Input: part model. Units: mm. Frame: model coordinates. A direction names the side the tool comes from. Round coordinates to 2 decimals unless told otherwise and drop trailing zeros. Order: outer loops, then holes, each group sorted by start corner. A loop starts at its lowest first (then second) coordinate and runs counter-clockwise, first axis right, second up. Notation, with made-up numbers: (89, 54.5) - (97, 54.5) arc R18 ccw to (97, 78.5) - close; hole circle Ø10 at (43.25, 60.5). An arc over 180 degrees is marked (long way). One line per item, written item: value. Start each with the question number.
from build123d import *

# Parameters (mm, degrees)
BOSS_EXTRUDE1_DEPTH   = 29
BOSS_EXTRUDE1_2_DEPTH = 29
FILLET1_R             = 1
FILLET2_R             = 1
SKETCH3_R             = 10
BOSS_EXTRUDE2_DEPTH   = 26.527316462
SKETCH4_R             = 2.5
CUT_EXTRUDE4_DEPTH    = 112.4075373


with BuildPart() as part:
    # Sketch1 → Boss-Extrude1 (new body)
    with BuildSketch(Plane.XY):
        with BuildLine():
            Line((-12.418786495, 106.527316462), (12.418786495, 106.527316462))
            ThreePointArc((12.418786495, 106.527316462), (14.186553448, 105.795083415), (14.918786495, 104.027316462))
            Line((14.918786495, 104.027316462), (14.918786495, 69.027316462))
            ThreePointArc((14.918786495, 69.027316462), (14.186553448, 67.259549509), (12.418786495, 66.527316462))
            Line((12.418786495, 66.527316462), (7.418786495, 66.527316462))
            Line((7.418786495, 66.527316462), (-7.418786495, 66.527316462))
            Line((-7.418786495, 66.527316462), (-12.418786495, 66.527316462))
            ThreePointArc((-12.418786495, 66.527316462), (-14.186553448, 67.259549509), (-14.918786495, 69.027316462))
            Line((-14.918786495, 69.027316462), (-14.918786495, 104.027316462))
            ThreePointArc((-14.918786495, 104.027316462), (-14.186553448, 105.795083415), (-12.418786495, 106.527316462))
        make_face()
    extrude(amount=BOSS_EXTRUDE1_DEPTH)

    # Fillet2
    fillet2_edges = [part.edges().sort_by_distance(p)[0] for p in [
        (14.186553448, 105.795083415, 0),
        (0, 106.527316462, 0),
        (-14.186553448, 105.795083415, 0),
        (-14.918786495, 86.527316462, 0),
        (-14.186553448, 67.259549509, 0),
        (0, 66.527316462, 0),
        (14.186553448, 67.259549509, 0),
        (14.918786495, 86.527316462, 0),
        (14.186553448, 105.795083415, 29),
        (0, 106.527316462, 29),
        (-14.186553448, 105.795083415, 29),
        (-14.918786495, 86.527316462, 29),
        (-14.186553448, 67.259549509, 29),
        (0, 66.527316462, 29),
        (14.186553448, 67.259549509, 29),
        (14.918786495, 86.527316462, 29),
    ]]
    fillet(fillet2_edges, radius=FILLET2_R)



with BuildPart() as body_2:
    # Sketch1 → Boss-Extrude1 2 (new body)
    with BuildSketch(Plane.XY):
        with BuildLine():
            Line((7.418786495, 40), (12.418786495, 40))
            ThreePointArc((12.418786495, 40), (14.186553448, 39.267766953), (14.918786495, 37.5))
            Line((14.918786495, 37.5), (14.918786495, -2.5))
            ThreePointArc((14.918786495, -2.5), (14.186553448, -4.267766953), (12.418786495, -5))
            Line((12.418786495, -5), (-12.418786495, -5))
            ThreePointArc((-12.418786495, -5), (-14.186553448, -4.267766953), (-14.918786495, -2.5))
            Line((-14.918786495, -2.5), (-14.918786495, 37.5))
            ThreePointArc((-14.918786495, 37.5), (-14.186553448, 39.267766953), (-12.418786495, 40))
            Line((-12.418786495, 40), (-7.418786495, 40))
            Line((-7.418786495, 40), (7.418786495, 40))
        make_face()
    extrude(amount=BOSS_EXTRUDE1_2_DEPTH)

    # Fillet1
    fillet1_edges = [body_2.edges().sort_by_distance(p)[0] for p in [
        (-14.918786495, 17.5, 0),
        (-14.186553448, 39.267766953, 0),
        (0, 40, 0),
        (14.186553448, 39.267766953, 0),
        (14.918786495, 17.5, 0),
        (14.186553448, -4.267766953, 29),
        (14.186553448, -4.267766953, 0),
        (0, -5, 0),
        (-14.186553448, -4.267766953, 0),
        (14.918786495, 17.5, 29),
        (14.186553448, 39.267766953, 29),
        (0, 40, 29),
        (-14.186553448, 39.267766953, 29),
        (-14.918786495, 17.5, 29),
        (-14.186553448, -4.267766953, 29),
        (0, -5, 29),
    ]]
    fillet(fillet1_edges, radius=FILLET1_R)


with BuildPart() as part_1:
    add(part.part)

    add(body_2.part)  # Boss-Extrude2 merges body 2
    # Sketch3 → Boss-Extrude2 (add)
    with BuildSketch(Plane(origin=(0, 40, 0), x_dir=(1, 0, 0), z_dir=(0, 1, 0))):
        with Locations(Location((0, -14.5, 0), (0, 0, 90))):
            Circle(SKETCH3_R)
    extrude(amount=BOSS_EXTRUDE2_DEPTH)

    # Sketch4 → Cut-Extrude4 (cut, through all)
    with BuildSketch(Plane(origin=(0, 0, 0), x_dir=(-1, 0, 0), z_dir=(0, 0, -1))):
        with Locations((0, 97.5)):
            Circle(SKETCH4_R)
        with Locations((0, 2.5)):
            Circle(SKETCH4_R)
    extrude(amount=-CUT_EXTRUDE4_DEPTH, mode=Mode.SUBTRACT)


solid = part_1.part
1. Section A-A (z = 26.25). Return the cut outline in (x, y), then the cut area to 3 significant figures.
2. Line query: line 1 (Y direction, x = 0, z = 15.25); line 2 (Y direction, x = -9.75, z = 9.75); line 3 (Y direction, x = -1.75, z = 11.75). Output: solid intervals per line, ascending. Write a range as from..to.
3. Section C-C (x = 0). Return the cut outline in (y, z).
4. Pull-direction query (Y, two-part tool) for faces 1 (the face through (-14.167, -4.287, 14.311)), 2 (the face through (-14.919, 86, 14)), 3 (the face through (-3, 53.08, 4.96)); classes: released by +Y, released by -Y, zero draft, split by the parting line, or undercut.
5. Set-up query: faces 4 (the face through (-14.206, 39.248, 14.311)), 5 (the face through (14.206, 67.279, 14.311)), 6 (the face through (8, 66.527, 8)). Return all of +Z, -Z, +X, -X, +Y, -Y with unobstructed straight access to the full face (end or side cutting, diameter ignored); none if empty.
6. Section D-D (z = 14.5). Return the cut outline in (x, y).
7. Pin query (flat end, axial travel): pin 1 (3 mm diameter, centred on y = 60.5, z = 8, fed in from -X); pin 2 (5 mm diameter, centred on y = 60, z = 17, fed in from -X); pin 3 (3 mm diameter, centred on x = 0, y = 2.5, fed in from -Z); pin 4 (5 mm diameter, centred on x = -0.5, y = 54, fed in from -Z). Return the tip coordinate at first contact, or that it passes through.
8. Section B-B (y = 2.5). Return the cut outline in (x, z), then the cut area to 3 significant figures.
Solved:
1. outline: (-14.92, -2.5) arc R2.5 ccw to (-12.42, -5) - (12.42, -5) arc R2.5 ccw to (14.92, -2.5) - (14.92, 37.5) arc R2.5 ccw to (12.42, 40) - (-12.42, 40) arc R2.5 ccw to (-14.92, 37.5) - close; (-14.92, 69.03) arc R2.5 ccw to (-12.42, 66.53) - (12.42, 66.53) arc R2.5 ccw to (14.92, 69.03) - (14.92, 104.03) arc R2.5 ccw to (12.42, 106.53) - (-12.42, 106.53) arc R2.5 ccw to (-14.92, 104.03) - close; hole circle Ø5 at (0, 2.5); hole circle Ø5 at (0, 97.5)
1. area: 2,490 mm²
2. line 1: y = -5..0, 5..95, 100..106.53
2. line 2: y = -5..40, 66.53..106.53
2. line 3: y = -5..0.71, 4.29..95.71, 99.29..106.53
3. outline: (-5, 1) arc R1 ccw to (-4, 0) - (0, 0) - (0, 29) - (-4, 29) arc R1 ccw to (-5, 28) - close; (5, 0) - (39, 0) arc R1 ccw to (40, 1) - (40, 4.5) - (66.53, 4.5) - (66.53, 1) arc R1 ccw to (67.53, 0) - (95, 0) - (95, 29) - (67.53, 29) arc R1 ccw to (66.53, 28) - (66.53, 24.5) - (40, 24.5) - (40, 28) arc R1 ccw to (39, 29) - (5, 29) - close; (100, 0) - (105.53, 0) arc R1 ccw to (106.53, 1) - (106.53, 28) arc R1 ccw to (105.53, 29) - (100, 29) - close
4. face 1: released by -Y
4. face 2: zero draft
4. face 3: undercut
5. face 4: +Z, -Z, -X
5. face 5: +Z, -Z, +X
5. face 6: none
6. outline: (-14.92, -2.5) arc R2.5 ccw to (-12.42, -5) - (12.42, -5) arc R2.5 ccw to (14.92, -2.5) - (14.92, 37.5) arc R2.5 ccw to (12.42, 40) - (10, 40) - (10, 66.53) - (12.42, 66.53) arc R2.5 ccw to (14.92, 69.03) - (14.92, 104.03) arc R2.5 ccw to (12.42, 106.53) - (-12.42, 106.53) arc R2.5 ccw to (-14.92, 104.03) - (-14.92, 69.03) arc R2.5 ccw to (-12.42, 66.53) - (-10, 66.53) - (-10, 40) - (-12.42, 40) arc R2.5 ccw to (-14.92, 37.5) - close; hole circle Ø5 at (0, 2.5); hole circle Ø5 at (0, 97.5)
7. pin 1: stops at x = -8.66
7. pin 2: stops at x = -10
7. pin 3: passes through
7. pin 4: stops at z = 4.5
8. outline: (-14.92, 1) arc R1 ccw to (-13.92, 0) - (-2.5, 0) - (-2.5, 29) - (-13.92, 29) arc R1 ccw to (-14.92, 28) - close; (2.5, 0) - (13.92, 0) arc R1 ccw to (14.92, 1) - (14.92, 28) arc R1 ccw to (13.92, 29) - (2.5, 29) - close
8. area: 719 mm²
